```python
from build123d import *

# Parameters (mm, degrees)
BOSS_EXTRUDE1_DEPTH = 2
SKETCH2_R           = 2.5
SKETCH2_R_2         = 3
CUT_EXTRUDE1_DEPTH  = 2


with BuildPart() as part:
    # Sketch1 → Boss-Extrude1 (new body)
    with BuildSketch(Plane.XY):
        with BuildLine():
            Line((0, 0), (30, 0))
            Line((30, 0), (30, 58))
            ThreePointArc((30, 58), (15, 73), (0, 58))
            Line((0, 58), (0, 0))
        make_face()
    extrude(amount=BOSS_EXTRUDE1_DEPTH)

    # Sketch2 → Cut-Extrude1 (cut)
    with BuildSketch(Plane.XY.offset(2)):
        with Locations((7.5, 10)):
            Circle(SKETCH2_R)
        with Locations((15, 58)):
            Circle(SKETCH2_R_2)
        with Locations((22.5, 10)):
            Circle(SKETCH2_R)
    extrude(amount=-CUT_EXTRUDE1_DEPTH, mode=Mode.SUBTRACT)


solid = part.part
```
Read the model definition and answer for the solid it produces. Units are mm, in the model's axes. Coordinates: 2 decimals unless noted, no trailing zeros. Write each loop counter-clockwise with the first axis right and the second up, starting at its lowest first coordinate (ties: lowest second). Pieces come first, ordered by that corner, then holes. Notation, with made-up numbers: (-27.75, -26.75) -> (22.25, -26.75) arc R9 ccw to (22.25, -17.75) -> close; hole circle Ø1 at (-38.5, 7.25). An arc over 180 degrees is marked (long way). Write item = value, one per line.
(1) Straight lines are drawn through the part: L1, parallel to Y at x = 15, z = 1.05; L2, parallel to Y at x = 7.5, z = 1.6; L3, parallel to X at y = 57, z = 0.6. For each, find the intervals that lie inside material, in ascending order. Write a range as from..to.
From the geometry:
L1 = 0..55, 61..73
L2 = 0..7.5, 12.5..70.99
L3 = 0..12.17, 17.83..30
(2) Section B-B on x = 15 is taken. Write down the section's boundary in (y, z).
From the geometry:
outline = (0, 0) -> (55, 0) -> (55, 2) -> (0, 2) -> close; (61, 0) -> (73, 0) -> (73, 2) -> (61, 2) -> close
(3) Section D-D on x = 22.5 is taken. Write down the section's boundary in (y, z).
From the geometry:
outline = (0, 0) -> (7.5, 0) -> (7.5, 2) -> (0, 2) -> close; (12.5, 0) -> (70.99, 0) -> (70.99, 2) -> (12.5, 2) -> close
(4) For a pull along Y with two mould halves and no side action, classify faces 1 (the face through (30, 29, 1)), 2 (the face through (15, 73, 1)), 3 (the face through (9, 8, 1)) as +Y half, -Y half, draft (parallel to the pull), parting line (faces both ways), or undercut.
From the geometry:
face_1 = draft
face_2 = +Y half
face_3 = undercut
(5) Section A-A on y = 10 is taken. Write down the section's boundary in (x, z), plus the area to 3 significant figures.
From the geometry:
outline = (0, 0) -> (5, 0) -> (5, 2) -> (0, 2) -> close; (10, 0) -> (20, 0) -> (20, 2) -> (10, 2) -> close; (25, 0) -> (30, 0) -> (30, 2) -> (25, 2) -> close
area = 40.0 mm2
(6) Section C-C on z = 1.4 is taken. Write down the section's boundary in (x, y), plus the area to 3 significant figures.
From the geometry:
outline = (0, 0) -> (30, 0) -> (30, 58) arc R15 ccw to (0, 58) -> close; hole circle Ø5 at (7.5, 10); hole circle Ø6 at (15, 58); hole circle Ø5 at (22.5, 10)
area = 2,030 mm2
